Part model, mm, in its own coordinate system. A direction names the side the tool comes from. Give positions to 0.01 mm unless a question says otherwise; leave off trailing zeros. Order: outer loops, then holes, each group sorted by start corner. A loop starts at its lowest first (then second) coordinate and runs counter-clockwise, first axis right, second up. Notation, with made-up numbers: M -38,4.5 L -30,4.5 A35 ccw -30,38.5 Z; hole C 21.5,26 d1. An arc over 180 degrees is marked long. Answer as a JSON object with one key per item and string values.
Autodesk Inventor part; units mm, degrees
ref_plane "YZ Plane" through (0, 0, 0) normal (1, 0, 0) x (0, 1, 0)
ref_plane "XZ Plane" through (0, 0, 0) normal (0, 1, 0) x (-1, 0, 0)
ref_plane "XY Plane" through (0, 0, 0) normal (0, 0, 1) x (1, 0, 0)
sketch "Sketch1" plane through (0, 0, 0) normal (0, 0, 1) x (1, 0, 0)
  line L0 (-19.05, 25.0245) -> (19.05, 25.0245)
  line L1 (19.05, 25.0245) -> (19.05, 44.0745)
  line L2 (19.05, 44.0745) -> (-19.05, 44.0745)
  line L3 (-19.05, 44.0745) -> (-19.05, 25.0245)
  line L4 (19.05, 56.7745) -> (25.4, 56.7745)
  line L5 (25.4, 56.7745) -> (25.4, 25.0245)
  line L6 (25.4, 25.0245) -> (19.05, 25.0245)
  line L7 (19.05, 25.0245) -> (19.05, 56.7745)
  line L8 (-19.05, 56.7745) -> (-25.4, 56.7745)
  line L9 (-25.4, 56.7745) -> (-25.4, 25.0245)
  line L10 (-25.4, 25.0245) -> (-19.05, 25.0245)
  line L11 (-19.05, 25.0245) -> (-19.05, 56.7745)
  line L12 (-27.7097, 23.437) -> (29.609, 23.437)
  point P0 (0, 0)
  dimension "d0" = 38.1
  dimension "d1" = 19.05
  dimension "d2" = 6.35
  dimension "d3" = 31.75
  dimension "d4" = 12.7
  dimension "d5" = 6.35
  dimension "d6" = 1.5875
  dimension "d8" = 31.75
revolve "Revolution1" add sketch "Sketch1" angle 360 about axis through (-27.7097, 23.437, 0) along (1, 0, 0)
properties part number "Spool"
1. Cut at A-A on y = 45.5. Give the cut face in (x, z).
Worked answers:
{"outline": "M -25.4,-24.99 L -19.05,-24.99 L -19.05,24.99 L -25.4,24.99 Z; M 19.05,-24.99 L 25.4,-24.99 L 25.4,24.99 L 19.05,24.99 Z"}
2. Two-plate mould, pull along X, no slides. Class faces 3 (the cylindrical face through (22.269, 55.235, 10.014)), 4 (the flat face through (-25.4, 23, -7)), 5 (the flat face through (19.05, 38, 15)): +X half, -X half, draft (parallel to the pull), parting line (faces both ways), or undercut.
Worked answers:
{"face 3": "draft", "face 4": "-X half", "face 5": "undercut"}
3. Pin check, flat tips, straight feed: P1, Ø4, axis at x = -20, y = 16, coming from the +Z side; P2, Ø12, axis at x = 2.5, y = 20, coming from the +Z side; P3, Ø1.5, axis at x = -1, z = 13.5, coming from the -Y side. Stop position of each tip, or through.
Worked answers:
{"P1": "stops at z = 32.89", "P2": "stops at z = 20.64", "P3": "stops at y = 7.21"}
4. Probe line 1 along X through (y, z) = (25.5, -24.5); line 2 along Z through (x, y) = (-6.5, 23.5); line 3 along Y through (x, z) = (19.5, -22). List the from-to ranges inside material, lowest first.
Worked answers:
{"line 1": "x = -25.4 to -19.05, 19.05 to 25.4", "line 2": "z = -20.64 to -1.59, 1.59 to 20.64", "line 3": "y = -1.61 to 48.48"}
5. Cut at B-B on z = 0. Give the cut face in (x, y), plus the area to 3 significant figures.
Worked answers:
{"outline": "M -25.4,-9.9 L -19.05,-9.9 L -19.05,2.8 L 19.05,2.8 L 19.05,-9.9 L 25.4,-9.9 L 25.4,21.85 L -25.4,21.85 Z; M -25.4,25.02 L 25.4,25.02 L 25.4,56.77 L 19.05,56.77 L 19.05,44.07 L -19.05,44.07 L -19.05,56.77 L -25.4,56.77 Z", "area": "2,260 mm^2"}
6. Which spindle directions (+Z, -Z, +X, -X, +Y, -Y) get a long thin tool onto all of the face, cutting with end or side? Do faces 1 (the flat face through (-19.05, 38, 15)), 2 (the cylindrical face through (0.36, 24.95, 0.48)). Say none if no direction does.
Worked answers:
{"face 1": "none", "face 2": "+X, -X"}
7. Cut at C-C on x = -5. Give the cut face in (y, z) (1 decimal), plus the area to 3 significant figures.
Worked answers:
{"outline": "C 23.4,0 d41.3; hole C 23.4,0 d3.2", "area": "1,330 mm^2"}
8. Cut at D-D on y = 7.5. Give the cut face in (x, z).
Worked answers:
{"outline": "M -25.4,-29.28 L -19.05,-29.28 L -19.05,-13.11 L 19.05,-13.11 L 19.05,-29.28 L 25.4,-29.28 L 25.4,29.28 L 19.05,29.28 L 19.05,13.11 L -19.05,13.11 L -19.05,29.28 L -25.4,29.28 Z"}
